```python
from build123d import *

# Parameters (mm, degrees)
SKETCH1_W               = 44.1
SKETCH1_H               = 44.1
BOSS_EXTRUDE1_DEPTH     = 10
SKETCH2_R               = 9.2
CUT_EXTRUDE1_DEPTH      = 8
SKETCH5_R               = 6.65
CUT_EXTRUDE4_DEPTH      = 50.9501001
MIRROR2_COPY_1_SKETCH_R = 9.2
MIRROR2_COPY_1_DEPTH    = 8
MIRROR2_COPY_2_SKETCH_R = 6.65
MIRROR2_COPY_2_DEPTH    = 50.9501001
CUT_EXTRUDE3_DEPTH      = 5


with BuildPart() as part:
    # Sketch1 → Boss-Extrude1 (new body)
    with BuildSketch(Plane(origin=(0, 0, 0), x_dir=(1, 0, 0), z_dir=(0, 1, 0))):
        with Locations((22.05, 0)):
            Rectangle(SKETCH1_W, SKETCH1_H)
    extrude(amount=BOSS_EXTRUDE1_DEPTH)

    # Sketch2 → Cut-Extrude1 (cut)
    with BuildSketch(Plane(origin=(0, 10, 0), x_dir=(1, 0, 0), z_dir=(0, 1, 0))):
        with Locations(Location((10.5, 11.55, 0), (0, 0, 270))):
            Circle(SKETCH2_R)
    cut_extrude1 = extrude(amount=-CUT_EXTRUDE1_DEPTH, mode=Mode.SUBTRACT)

    # Sketch5 → Cut-Extrude4 (cut, through all)
    with BuildSketch(Plane(origin=(0, 2, 0), x_dir=(1, 0, 0), z_dir=(0, 1, 0))):
        with Locations(Location((10.5, 11.55, 0), (0, 0, 270))):
            Circle(SKETCH5_R)
    cut_extrude4 = extrude(amount=-CUT_EXTRUDE4_DEPTH, mode=Mode.SUBTRACT)

    # Mirror1: Cut-Extrude1, Cut-Extrude4 across plane
    add(cut_extrude1.mirror(Plane.XY), mode=Mode.SUBTRACT)
    add(cut_extrude4.mirror(Plane.XY), mode=Mode.SUBTRACT)

    # Mirror2: Cut-Extrude1, Cut-Extrude4 across plane
    add(cut_extrude1.mirror(Plane(origin=(22.05, 0, 0), x_dir=(0, 0, 1), z_dir=(1, 0, 0))), mode=Mode.SUBTRACT)
    add(cut_extrude4.mirror(Plane(origin=(22.05, 0, 0), x_dir=(0, 0, 1), z_dir=(1, 0, 0))), mode=Mode.SUBTRACT)

    # Mirror2 copy 1 sketch → Mirror2 copy 1 (cut)
    with BuildSketch(Plane(origin=(44.1, 10, 0), x_dir=(-1, 0, 0), z_dir=(0, 1, 0))):
        with Locations(Location((10.5, 11.55, 0), (0, 0, 270))):
            Circle(MIRROR2_COPY_1_SKETCH_R)
    extrude(amount=-MIRROR2_COPY_1_DEPTH, mode=Mode.SUBTRACT)

    # Mirror2 copy 2 sketch → Mirror2 copy 2 (cut, through all)
    with BuildSketch(Plane(origin=(44.1, 2, 0), x_dir=(-1, 0, 0), z_dir=(0, 1, 0))):
        with Locations(Location((10.5, 11.55, 0), (0, 0, 270))):
            Circle(MIRROR2_COPY_2_SKETCH_R)
    extrude(amount=-MIRROR2_COPY_2_DEPTH, mode=Mode.SUBTRACT)

    # Sketch4 → Cut-Extrude3 (cut)
    with BuildSketch(Plane(origin=(0, 10, 0), x_dir=(1, 0, 0), z_dir=(0, 1, 0))):
        Polygon((21.05, 22.05), (23.05, 22.05), (23.05, 1), (46.251393124, 1), (46.251393124, -1), (23.05, -1), (23.05, -23.362709558), (21.05, -23.362709558), (21.05, -1), (0, -1), (0, 1), (21.05, 1), align=None)
    extrude(amount=-CUT_EXTRUDE3_DEPTH, mode=Mode.SUBTRACT)


solid = part.part
```
Build history of the part. All positions in model axes, mm. A direction names the side the tool comes from. Give positions to 0.01 mm unless a question says otherwise; leave off trailing zeros. Order: outer loops, then holes, each group sorted by start corner. A loop starts at its lowest first (then second) coordinate and runs counter-clockwise, first axis right, second up. Notation, with made-up numbers: M 1,-26 L 38,-26 A31 ccw 38,11 Z; hole C 15,-16.75 d9. An arc over 180 degrees is marked long. Write item = value, one per line. Start each with the question number.
(1) Slice it at B-B on x = 33.6. Write the cut outline in (y, z), plus the area to 3 significant figures.
(2) Probe L1, parallel to X at y = 8.5, z = -12; L2, parallel to X at y = 4.75, z = -11.55; L3, parallel to X at y = 1.55, z = -11.55. List the from-to ranges inside material, lowest first. Write a range as [from, to].
(3) Slice it at A-A on y = 6.5. Write the cut outline in (x, z).
(4) Slice it at C-C on z = 11.55. Write the cut outline in (x, y).
(5) Pin check, flat tips, straight feed: pin 1 Ø11 at (x, z) = (10.5, 11.55) entering from +Y; pin 2 Ø9 at (x, z) = (34, 14.5) entering from +Y. Stop position of each tip, or through.
(6) Which spindle directions (+Z, -Z, +X, -X, +Y, -Y) get a long thin tool onto all of the face, cutting with end or side? Do faces 1 (the flat face through (0, 4, 0)), 2 (the flat face through (33, 8, -1)), 3 (the flat face through (21.05, 8, -11)), 4 (the flat face through (40, 2, 9)). Say none if no direction does.
(7) Two-plate mould, pull along Z, no slides. Class faces 5 (the flat face through (10, 10, 2)), 6 (the flat face through (22, 5, 0)): released by +Z, released by -Z, zero draft, split by the parting line, or undercut.
Responses:
q1.outline = M 0,-22.05 L 10,-22.05 L 10,-20.75 L 2,-20.75 L 2,-18.2 L 0,-18.2 Z; M 0,-4.9 L 2,-4.9 L 2,-2.35 L 10,-2.35 L 10,-1 L 5,-1 L 5,1 L 10,1 L 10,2.35 L 2,2.35 L 2,4.9 L 0,4.9 Z; M 0,18.2 L 2,18.2 L 2,20.75 L 10,20.75 L 10,22.05 L 0,22.05 Z
q1.area = 83.4 mm2
q2.L1 = [0, 1.31], [19.69, 21.05], [23.05, 24.41], [42.79, 44.1]
q2.L2 = [0, 1.3], [19.7, 24.4], [42.8, 44.1]
q2.L3 = [0, 3.85], [17.15, 26.95], [40.25, 44.1]
q3.outline = M 0,-22.05 L 21.05,-22.05 L 21.05,-1 L 0,-1 Z; M 0,1 L 21.05,1 L 21.05,22.05 L 0,22.05 Z; M 23.05,-22.05 L 44.1,-22.05 L 44.1,-1 L 23.05,-1 Z; M 23.05,1 L 44.1,1 L 44.1,22.05 L 23.05,22.05 Z; hole C 10.5,-11.55 d18.4; hole C 10.5,11.55 d18.4; hole C 33.6,-11.55 d18.4; hole C 33.6,11.55 d18.4
q4.outline = M 0,0 L 3.85,0 L 3.85,2 L 1.3,2 L 1.3,10 L 0,10 Z; M 17.15,0 L 26.95,0 L 26.95,2 L 24.4,2 L 24.4,10 L 23.05,10 L 23.05,5 L 21.05,5 L 21.05,10 L 19.7,10 L 19.7,2 L 17.15,2 Z; M 40.25,0 L 44.1,0 L 44.1,10 L 42.8,10 L 42.8,2 L 40.25,2 Z
q5.pin_1 = through
q5.pin_2 = 2
q6.face_1 = +Z, -Z, -X, +Y, -Y
q6.face_2 = +X, -X, +Y
q6.face_3 = +Z, -Z, +Y
q6.face_4 = +Y
q7.face_5 = zero draft
q7.face_6 = undercut
